from build123d import *

# Parameters (mm, degrees)
BOSS_EXTRUDE1_DEPTH      = 37.5
BOSS_EXTRUDE1_DEPTH_BACK = 28
CUT_EXTRUDE2_START       = -28
CUT_EXTRUDE2_DEPTH       = 18
CUT_EXTRUDE3_START       = 10
CUT_EXTRUDE3_DEPTH       = 27.5
SKETCH6_OUTSIDE_W        = 110.594
SKETCH6_OUTSIDE_H        = 74.594
CUT_EXTRUDE4_DEPTH       = 8
SKETCH7_OUTSIDE_W        = 110.594
SKETCH7_OUTSIDE_H        = 74.594
SKETCH7_OUTSIDE_R        = 14
CUT_EXTRUDE5_DEPTH       = 3


# Read off the part's stored shape, not the designer's step: Cut-Extrude2, Cut-Extrude3
with BuildPart() as part:
    # Sketch1 → Boss-Extrude1 (new, two sides: drawn at the far end of the back side and taken through both)
    with BuildSketch(Plane.XY.offset(-BOSS_EXTRUDE1_DEPTH_BACK)):
        with BuildLine():
            Line((-42.5, 2.3), (-40.572637014, 2.3))
            Line((-40.572637014, 2.3), (-41.319077862, 4.350829376))
            ThreePointArc((-41.319077862, 4.350829376), (-41.136451338, 6.808366086), (-39.174853163, 8.3))
            Line((-39.174853163, 8.3), (-10.741593286, 14.864335276))
            ThreePointArc((-10.741593286, 14.864335276), (-8.862822134, 15.738832848), (-7.5, 17.3))
            Line((-7.5, 17.3), (7.5, 17.3))
            ThreePointArc((7.5, 17.3), (8.862822134, 15.738832848), (10.741593286, 14.864335276))
            Line((10.741593286, 14.864335276), (39.174853163, 8.3))
            ThreePointArc((39.174853163, 8.3), (41.136451338, 6.808366086), (41.319077862, 4.350829376))
            Line((41.319077862, 4.350829376), (40.572637014, 2.3))
            Line((40.572637014, 2.3), (42.5, 2.3))
            Line((42.5, 2.3), (42.5, -31.7))
            Line((42.5, -31.7), (-42.5, -31.7))
            Line((-42.5, -31.7), (-42.5, 2.3))
        make_face()
    extrude(amount=BOSS_EXTRUDE1_DEPTH + BOSS_EXTRUDE1_DEPTH_BACK)

    # Sketch2 → Cut-Revolve1 (revolve, cut)
    with BuildSketch(Plane(origin=(0, 0, 0), x_dir=(0, 0, -1), z_dir=(1, 0, 0))):
        with BuildLine():
            Line((-3.5, -125), (-3.5, 0))
            ThreePointArc((-3.5, 0), (0, 3.5), (3.5, 0))
            Line((3.5, 0), (3.5, -125))
            Line((3.5, -125), (-3.5, -125))
        make_face()
    revolve(axis=Axis((0, -125, 37.5), (0, 0, -1)), mode=Mode.SUBTRACT)

    # Cut-Extrude2 outline → Cut-Extrude2 (cut)
    with BuildSketch(Plane.XY.offset(CUT_EXTRUDE2_START)):
        with BuildLine():
            ThreePointArc((7.5, 12.3), (10.428932188, 5.228932188), (17.5, 2.3))
            Line((17.5, 2.3), (40.572637014, 2.3))
            Line((40.572637014, 2.3), (41.319077862, 4.350829376))
            ThreePointArc((41.319077862, 4.350829376), (41.136451338, 6.808366087), (39.174853163, 8.3))
            Line((39.174853163, 8.3), (10.741593286, 14.864335276))
            ThreePointArc((10.741593286, 14.864335276), (8.862822134, 15.738832848), (7.5, 17.3))
            Line((7.5, 17.3), (7.5, 12.3))
        make_face()
        with BuildLine():
            Line((-41.319077862, 4.350829376), (-40.572637014, 2.3))
            Line((-40.572637014, 2.3), (-17.5, 2.3))
            ThreePointArc((-17.5, 2.3), (-10.428932188, 5.228932188), (-7.5, 12.3))
            Line((-7.5, 12.3), (-7.5, 17.3))
            ThreePointArc((-7.5, 17.3), (-8.862822134, 15.738832848), (-10.741593286, 14.864335276))
            Line((-10.741593286, 14.864335276), (-39.174853163, 8.3))
            ThreePointArc((-39.174853163, 8.3), (-41.136451338, 6.808366087), (-41.319077862, 4.350829376))
        make_face()
    extrude(amount=CUT_EXTRUDE2_DEPTH, mode=Mode.SUBTRACT)

    # Cut-Extrude3 outline → Cut-Extrude3 (cut)
    with BuildSketch(Plane.XY.offset(CUT_EXTRUDE3_START)):
        with BuildLine():
            ThreePointArc((7.5, 12.3), (10.428932188, 5.228932188), (17.5, 2.3))
            Line((17.5, 2.3), (40.572637014, 2.3))
            Line((40.572637014, 2.3), (41.319077862, 4.350829376))
            ThreePointArc((41.319077862, 4.350829376), (41.136451338, 6.808366087), (39.174853163, 8.3))
            Line((39.174853163, 8.3), (10.741593286, 14.864335276))
            ThreePointArc((10.741593286, 14.864335276), (8.862822134, 15.738832848), (7.5, 17.3))
            Line((7.5, 17.3), (7.5, 12.3))
        make_face()
        with BuildLine():
            Line((-41.319077862, 4.350829376), (-40.572637014, 2.3))
            Line((-40.572637014, 2.3), (-17.5, 2.3))
            ThreePointArc((-17.5, 2.3), (-10.428932188, 5.228932188), (-7.5, 12.3))
            Line((-7.5, 12.3), (-7.5, 17.3))
            ThreePointArc((-7.5, 17.3), (-8.862822134, 15.738832848), (-10.741593286, 14.864335276))
            Line((-10.741593286, 14.864335276), (-39.174853163, 8.3))
            ThreePointArc((-39.174853163, 8.3), (-41.136451338, 6.808366087), (-41.319077862, 4.350829376))
        make_face()
    extrude(amount=CUT_EXTRUDE3_DEPTH, mode=Mode.SUBTRACT)

    # Sketch5 → Cut-Revolve2 (revolve, cut)
    with BuildSketch(Plane.XY.offset(21), mode=Mode.PRIVATE) as cut_revolve2_sk:
        Polygon((-35, -31.7), (-40, -31.7), (-40, -28.7), (-39, -28.7), (-39, 17.3), (-35, 17.3), align=None)
    cut_revolve2 = revolve(cut_revolve2_sk.sketch.rotate(Axis((-35, -31.7, 21), (0, 1, 0)), 270), axis=Axis((-35, -31.7, 21), (0, 1, 0)), mode=Mode.SUBTRACT)

    # Mirror1: Cut-Revolve2 across plane
    add(cut_revolve2.mirror(Plane(origin=(0, 0, 0), x_dir=(0, 0, 1), z_dir=(1, 0, 0))), mode=Mode.SUBTRACT)

    # Sketch6 outside → Cut-Extrude4 (cut)
    with BuildSketch(Plane.XY.offset(37.5)):
        with Locations((0, -7.2)):
            Rectangle(SKETCH6_OUTSIDE_W, SKETCH6_OUTSIDE_H)
        with BuildLine():
            Line((20.5, 2.3), (11.489125293, 2.3))
            ThreePointArc((11.489125293, 2.3), (7.785844894, 3.208757917), (4.92391084, 5.728571429))
            ThreePointArc((4.92391084, 5.728571429), (0, 8.3), (-4.92391084, 5.728571429))
            ThreePointArc((-4.92391084, 5.728571429), (-7.785844894, 3.208757917), (-11.489125293, 2.3))
            Line((-11.489125293, 2.3), (-20.5, 2.3))
            ThreePointArc((-20.5, 2.3), (-37.5, -14.7), (-20.5, -31.7))
            Line((-20.5, -31.7), (20.5, -31.7))
            ThreePointArc((20.5, -31.7), (37.5, -14.7), (20.5, 2.3))
        make_face(mode=Mode.SUBTRACT)
    extrude(amount=-CUT_EXTRUDE4_DEPTH, mode=Mode.SUBTRACT)

    # Sketch7 outside → Cut-Extrude5 (cut)
    with BuildSketch(Plane.XY.offset(37.5)):
        with Locations((0, -7.2)):
            Rectangle(SKETCH7_OUTSIDE_W, SKETCH7_OUTSIDE_H)
        with Locations((-20.5, -14.7)):
            Circle(SKETCH7_OUTSIDE_R, mode=Mode.SUBTRACT)
        with Locations((20.5, -14.7)):
            Circle(SKETCH7_OUTSIDE_R, mode=Mode.SUBTRACT)
    extrude(amount=-CUT_EXTRUDE5_DEPTH, mode=Mode.SUBTRACT)

    # Sketch8 → Revolve1 (revolve)
    with BuildSketch(Plane.XY.offset(-15.75)):
        Polygon((-56, -14.7), (-56, -17.45), (-55, -17.45), (-55, -17.2), (-48.5, -17.2), (-48.5, -19.7), (-42.5, -19.7), (-42.5, -14.7), align=None)
        Polygon((42.5, -19.7), (42.5, -14.7), (56, -14.7), (56, -17.45), (55, -17.45), (55, -17.2), (48.5, -17.2), (48.5, -19.7), align=None)
    revolve(axis=Axis((-56, -14.7, -15.75), (1, 0, 0)))


solid = part.part
The model under review builds one solid part; all positions refer to its coordinate system, in mm. A direction names the side the tool comes from. Coordinates: 2 decimals unless noted, no trailing zeros. Write each loop counter-clockwise with the first axis right and the second up, starting at its lowest first coordinate (ties: lowest second). Pieces come first, ordered by that corner, then holes. Notation, with made-up numbers: (86.25, 20) -> (136.25, 20) arc R9 ccw to (136.25, 36) -> close; hole circle Ø5 at (25.25, 42). An arc over 180 degrees is marked (long way). Answer in a Markdown table with one row per item.
1. For faces 4 (the flat face through (-21, 8, 10)), 5 (the cylindrical face through (-55.493, -14.342, -18.477)), 6 (the cylindrical face through (-51.7, -14.2, -13.3)), 7 (the flat face through (1, -16, -3.5)), 8 (the flat face through (24, 8, -10)), list the 3-axis set-ups (+Z, -Z, +X, -X, +Y, -Y) from which the entire face can be reached by the end or side of a thin tool; tool diameter is ignored.
Answers below:
| item | result |
|---|---|
| face 4 | +Z, -X, +Y |
| face 5 | -X |
| face 6 | none |
| face 7 | -Y |
| face 8 | -Z, +X, +Y |
2. We need section D-D, the plane x = 45.5. State the section outline as (y, z) points, and give its area (3 significant figures).
Answers below:
| item | result |
|---|---|
| outline | circle Ø10 at (-14.7, -15.75) |
| area | 78.5 mm^2 |
3. We need section A-A, the plane z = 21. State the section outline as (x, y) points.
Answers below:
| item | result |
|---|---|
| outline | (-42.5, -31.7) -> (-40, -31.7) -> (-40, -28.7) -> (-39, -28.7) -> (-39, 2.3) -> (-42.5, 2.3) -> close; (-31, -28.7) -> (-30, -28.7) -> (-30, -31.7) -> (30, -31.7) -> (30, -28.7) -> (31, -28.7) -> (31, 2.3) -> (17.5, 2.3) arc R10 cw to (7.5, 12.3) -> (7.5, 17.3) -> (-7.5, 17.3) -> (-7.5, 12.3) arc R10 cw to (-17.5, 2.3) -> (-31, 2.3) -> close; (39, -28.7) -> (40, -28.7) -> (40, -31.7) -> (42.5, -31.7) -> (42.5, 2.3) -> (39, 2.3) -> close |
4. Clearance check with flat-ended pins moving along their axes: pin 1 Ø3 at (y, z) = (11.5, -16) entering from -X; pin 2 Ø2 at (y, z) = (-12.5, 28.5) entering from -X; pin 3 Ø1.5 at (x, y) = (15.5, 6) entering from +Z. State where each tip first meets the part, or that it passes through.
Answers below:
| item | result |
|---|---|
| pin 1 | stops at x = -7.77 |
| pin 2 | stops at x = -42.5 |
| pin 3 | stops at z = 10 |
5. Wall thickness on probe 1 along Z at (x, y) = (-35, -29.5); probe 2 along Z at (x, y) = (24.5, -21.5); probe 3 along Z at (x, y) = (40, -22.5): over which ranges is each line inside the solid? List them lowest first. Write a range as [from, to].
Answers below:
| item | result |
|---|---|
| probe 1 | z = [-28, -3.5], [3.5, 16], [26, 29.5] |
| probe 2 | z = [-28, -3.5], [3.5, 37.5] |
| probe 3 | z = [-28, -3.5], [3.5, 29.5] |
6. Draft analysis for pull direction X (two halves, no side actions). For faces 1 (the flat face through (0, -13, 34.5)), 2 (the flat face through (1, -31.7, -16)), 3 (the flat face through (-7.5, 15, 20)), state which applies: +X half, -X half, draft (parallel to the pull), parting line (faces both ways), or undercut.
Answers below:
| item | result |
|---|---|
| face 1 | undercut |
| face 2 | draft |
| face 3 | -X half |
7. We need section B-B, the plane y = -21. State the section outline as (x, z) points.
Answers below:
| item | result |
|---|---|
| outline | (-42.5, -28) -> (42.5, -28) -> (42.5, -3.5) -> (-42.5, -3.5) -> close; (-42.5, 3.5) -> (42.5, 3.5) -> (42.5, 29.5) -> (36.29, 29.5) -> (36.29, 34.5) -> (33, 34.5) -> (33, 37.5) -> (8, 37.5) -> (8, 34.5) -> (-8, 34.5) -> (-8, 37.5) -> (-33, 37.5) -> (-33, 34.5) -> (-36.29, 34.5) -> (-36.29, 29.5) -> (-42.5, 29.5) -> close; hole circle Ø8 at (-35, 21); hole circle Ø8 at (35, 21) |
